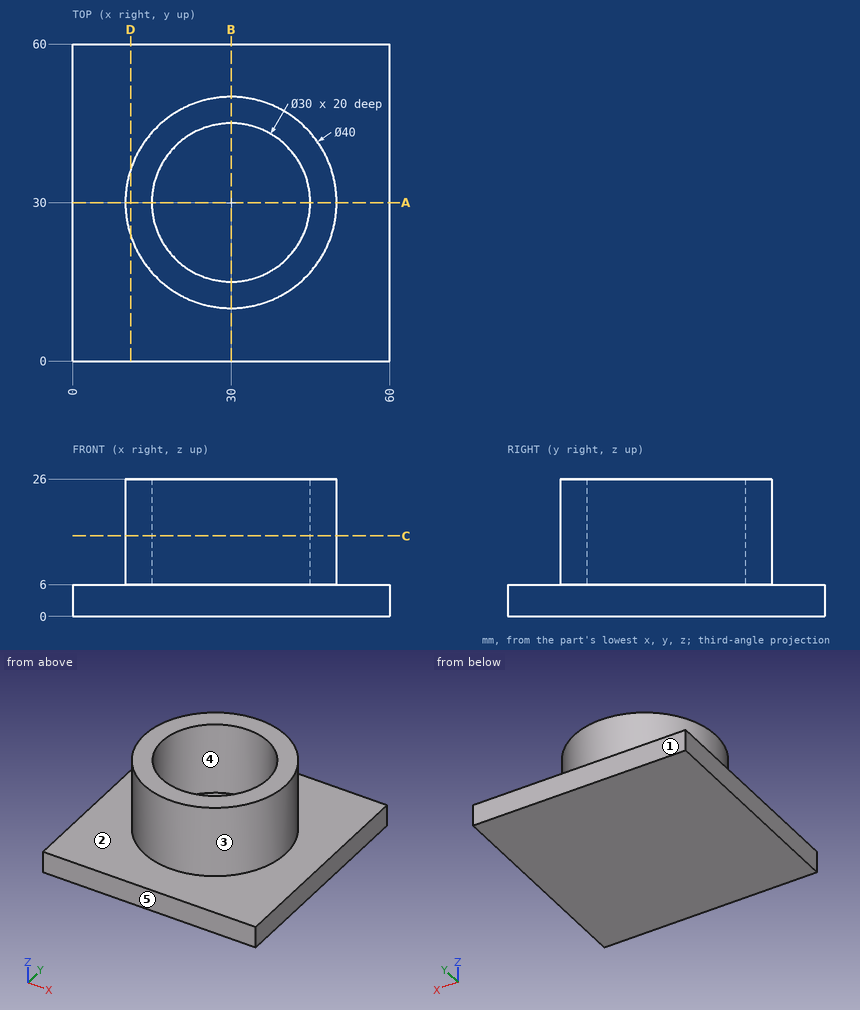
The drawing under review shows one solid part. Ordinate dimensions are in mm from its lowest x, y, z. A direction names the side the tool comes from. Coordinates: 2 decimals unless noted, no trailing zeros. Write each loop counter-clockwise with the first axis right and the second up, starting at its lowest first coordinate (ties: lowest second). Pieces come first, ordered by that corner, then holes. Notation, with made-up numbers: (-17, -38.5) - (38, -38.5) arc R19 ccw to (38, -9.5) - close; hole circle Ø9 at (-10.75, -9). An arc over 180 degrees is marked (long way). Answer as CSV lines item,"result".
(1) Clearance check with flat-ended pins moving along their axes: pin 1 Ø2 at (y, z) = (43.5, 8.5) entering from -X; pin 2 Ø1 at (x, z) = (17.5, 8.5) entering from +Y; pin 3 Ø3 at (x, z) = (12.5, 19) entering from -Y; pin 4 Ø2 at (x, y) = (7.5, 51) entering from -Z. State where each tip first meets the part, or that it passes through.
Data:
pin 1,"stops at x = 14.39"
pin 2,"stops at y = 46"
pin 3,"stops at y = 18"
pin 4,"stops at z = 0"
(2) Tool access review of the marked faces 1 and 2: name each direction out of +Z, -Z, +X, -X, +Y, -Y from which nothing blocks a thin tool from reaching the whole face with its end or side.
Data:
face 1,"+Z, -Z, +X, -X, +Y"
face 2,"+Z"
(3) We need section C-C (z = 15.25). Give the boundary of the cut face in (x, y), plus the area to 3 significant figures.
Data:
outline,"circle Ø40 at (30, 30); hole circle Ø30 at (30, 30)"
area,"550 mm2"
(4) Mouldability with a two-part tool opening along X and no side actions: class the marked faces 3, 4 and 5 as pulls with the +X half, pulls with the -X half, needs draft (parallel to the pull), parting line crosses it, or undercut.
Data:
face 3,"parting line crosses it"
face 4,"undercut"
face 5,"needs draft"
(5) We need section D-D (x = 11). Give the boundary of the cut face in (y, z) (3 decimals), plus the area to 3 significant figures.
Data:
outline,"(0, 0) - (60, 0) - (60, 6) - (36.245, 6) - (36.245, 26) - (23.755, 26) - (23.755, 6) - (0, 6) - close"
area,"610 mm2"
(6) We need section A-A (y = 30). Give the boundary of the cut face in (x, z).
Data:
outline,"(0, 0) - (60, 0) - (60, 6) - (50, 6) - (50, 26) - (45, 26) - (45, 6) - (15, 6) - (15, 26) - (10, 26) - (10, 6) - (0, 6) - close"
(7) For line 1 along Y through (x, z) = (30, 14); line 2 along Z through (x, y) = (55, 35.5); line 3 along Y through (x, z) = (23.5, 19.5), list the stretches that pass through material, from the lowest coordinate up. Write a range as [from, to].
Data:
line 1,"y = [10, 15], [45, 50]"
line 2,"z = [0, 6]"
line 3,"y = [11.09, 16.48], [43.52, 48.91]"
